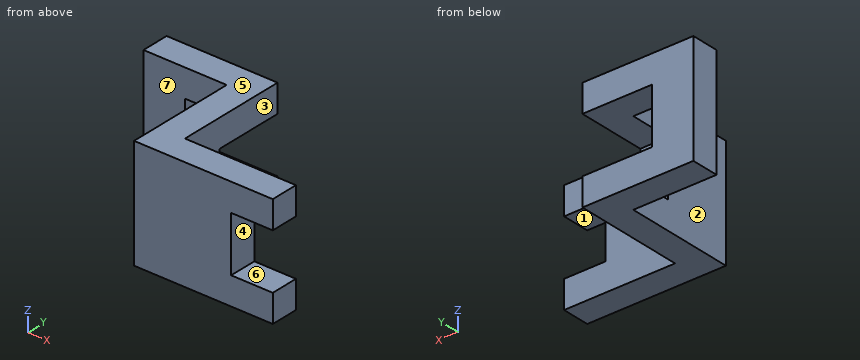
from build123d import *

# Parameters (mm, degrees)
BOSS_EXTRUDE3_DEPTH     = 40
CUT_EXTRUDE1_DEPTH      = 1
CUT_EXTRUDE1_DEPTH_BACK = 25
CUT_EXTRUDE2_DEPTH      = 11


with BuildPart() as part:
    # Sketch4 → Boss-Extrude3 (new body)
    with BuildSketch(Plane.XY):
        Polygon((0, 0), (0, -10), (30, -10), (30, -50), (80, -50), (80, -40), (40, -40), (40, 0), align=None)
    extrude(amount=BOSS_EXTRUDE3_DEPTH)

    # Sketch5 → Cut-Extrude1 (cut, two sides)
    with BuildSketch(Plane(origin=(0, 0, 0), x_dir=(1, 0, 0), z_dir=(0, 1, 0))) as cut_extrude1_sk:
        Polygon((150, -10), (40, -10), (15, -10), (15, -30), (40, -30), (150, -30), (370, -30), (370, -10), align=None)
    extrude(amount=CUT_EXTRUDE1_DEPTH, mode=Mode.SUBTRACT)
    extrude(cut_extrude1_sk.sketch, amount=-CUT_EXTRUDE1_DEPTH_BACK, mode=Mode.SUBTRACT)

    # Sketch6 → Cut-Extrude2 (cut, through all)
    with BuildSketch(Plane(origin=(0, -40, 0), x_dir=(1, 0, 0), z_dir=(0, 1, 0))):
        Polygon((260.880074906, -10), (80, -10), (65, -10), (65, -30), (80, -30), (260.880074906, -30), (622.640224719, -30), (622.640224719, -10), align=None)
    extrude(amount=-CUT_EXTRUDE2_DEPTH, mode=Mode.SUBTRACT)


solid = part.part
Design review of the part built by this model. Coordinates are the model's own, in mm. Face numbers are marked on the shaded views. A direction names the side the tool comes from. Give positions to 0.01 mm unless a question says otherwise; leave off trailing zeros. Write each loop counter-clockwise with the first axis right and the second up, starting at its lowest first coordinate (ties: lowest second). Pieces come first, ordered by that corner, then holes. Notation, with made-up numbers: M -8,-31 L 5,-31 A31 cw 5,-3 Z; hole C -31,53.5 d5. An arc over 180 degrees is marked long. Answer as a JSON object with one key per item and string values. Group by question number.
1) We need section C-C (x = 32). Give the boundary of the cut face in (y, z), and give its area (3 significant figures).
2) Clearance check with flat-ended pins moving along their axes: pin 1 Ø5 at (y, z) = (-11, 9.5) entering from +X; pin 2 Ø15 at (x, z) = (15.5, 15) entering from -Y; pin 3 Ø20 at (x, z) = (61, 28.5) entering from +Y; pin 4 Ø2 at (y, z) = (-20.5, 12) entering from -X (3 decimals). State where each tip first meets the part, or that it passes through.
3) We need section B-B (y = -45.5). Give the boundary of the cut face in (x, z), and give its area (3 significant figures).
4) We need section D-D (y = -19.5). Give the boundary of the cut face in (x, z), and give its area (3 significant figures).
5) Mouldability with a two-part tool opening along Z and no side actions: class the marked faces 4, 5, 6 and 7 as released by +Z, released by -Z, zero draft, split by the parting line, or undercut.
6) We need section A-A (z = 21.5). Give the boundary of the cut face in (x, y).
7) Tool access review of the marked faces 1, 2 and 3: name each direction out of +Z, -Z, +X, -X, +Y, -Y from which nothing blocks a thin tool from reaching the whole face with its end or side.
8) For line 1 along Z through (x, y) = (17, -2.5); line 2 along Y through (x, z) = (15.5, 36.5); line 3 along Y through (x, z) = (41, 23.5), list the stretches that pass through material, from the lowest coordinate up.
Answer key:
{
 "1": {"outline": "M -50,0 L 0,0 L 0,10 L -25,10 L -25,30 L 0,30 L 0,40 L -50,40 Z", "area": "1,500 mm²"},
 "2": {"pin 1": "stops at x = 40", "pin 2": "stops at y = -10", "pin 3": "stops at y = -40", "pin 4": "passes through"},
 "3": {"outline": "M 30,0 L 80,0 L 80,10 L 65,10 L 65,30 L 80,30 L 80,40 L 30,40 Z", "area": "1,700 mm²"},
 "4": {"outline": "M 30,0 L 40,0 L 40,10 L 30,10 Z; M 30,30 L 40,30 L 40,40 L 30,40 Z", "area": "200 mm²"},
 "5": {"face 4": "undercut", "face 5": "released by +Z", "face 6": "undercut", "face 7": "zero draft"},
 "6": {"outline": "M 0,-10 L 15,-10 L 15,0 L 0,0 Z; M 30,-50 L 65,-50 L 65,-40 L 40,-40 L 40,-25 L 30,-25 Z"},
 "7": {"face 1": "+X, +Y, -Y", "face 2": "+Z, -Z, -X, -Y", "face 3": "+Z, -Z, +X, +Y"},
 "8": {"line 1": "z = 0 to 10, 30 to 40", "line 2": "y = -10 to 0", "line 3": "y = -50 to -40"}
}
